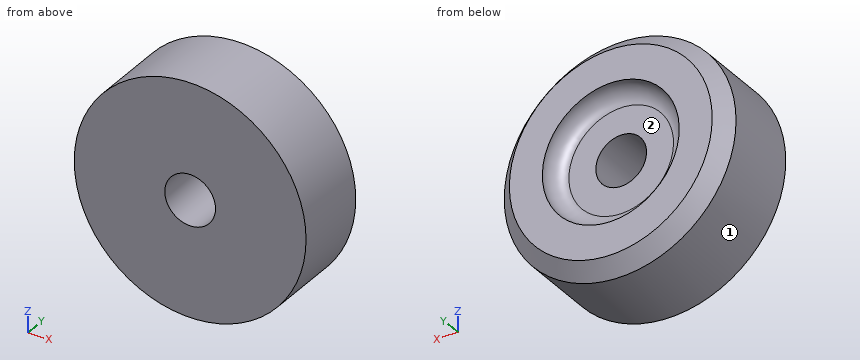
Autodesk Inventor part; units mm, degrees
ref_plane "YZ Plane" through (0, 0, 0) normal (1, 0, 0) x (0, 1, 0)
ref_plane "XZ Plane" through (0, 0, 0) normal (0, 1, 0) x (-1, 0, 0)
ref_plane "XY Plane" through (0, 0, 0) normal (0, 0, 1) x (1, 0, 0)
sketch "Sketch1" plane through (0, 0, 0) normal (0, 0, 1) x (1, 0, 0)
  line L0 (0, 0) -> (0, 6.35)
  line L1 (12.7, 0) -> (0, 0)
  circle A0 centre (10.1178, 6.9428) radius 1.5875
  line L2 (0, 6.35) -> (8.6451, 6.35)
  line L3 (12.7, 0) -> (12.7, 6.35)
  line L4 (12.7, 6.35) -> (11.5905, 6.35)
  line L5 (9.525, 8.4155) -> (0, 8.4155)
  line L6 (0, 8.4155) -> (0, 6.35)
  line L7 (9.525, 8.4155) -> (11.5905, 6.35) construction
  line L8 (9.525, 8.4155) -> (9.525, 10.003)
  line L9 (9.525, 10.003) -> (0, 10.003)
  line L10 (0, 10.003) -> (0, 8.4155)
  line L11 (12.7, 6.35) -> (12.7, 10.003)
  line L12 (12.7, 10.003) -> (9.525, 10.003)
  dimension "d0" = 3.175
  dimension "d5" = 45
  dimension "d6" = 1.5875
  dimension "d7" = 3.175
  dimension "d8" = 6.35
  dimension "d14" = 2.921
  dimension "d37" = 12.7
revolve "Revolution1" add sketch "Sketch1" angle 360 about axis through (0, 10.003, 0) along (0, -1, 0)
sketch "Sketch8" plane through (0, 0, 0) normal (1, 0, 0) x (0, 1, 0)
  circle A0 centre (10.003, -5.734) radius 1.7653
  line L0 (10.003, 0) -> (8.2377, 0)
  line L1 (8.2377, 0) -> (8.2377, -5.734)
  line L2 (10.003, 13.6947) -> (10.003, -13.6947)
  line L3 (10.003, -5.734) -> (10.003, -3.9688) construction
  line L4 (-2.3537, 0) -> (14.1219, 0)
  point P0 (0, 0)
  dimension "d31" = 3.5306
  dimension "d32" = 3.9688
revolve "Revolution3" cut sketch "Sketch8" angle 360 about axis through (0, -10, 0) along (0, 1, 0)
sketch "Sketch9" plane through (0, 8.2377, 0) normal (0, 1, 0) x (1, 0, 0)
  circle A0 centre (0, 0) radius 2.7781
  dimension "d34" = 5.5563
extrude "Extrusion4" cut sketch "Sketch9" against normal through all
chamfer "Chamfer3" distance 1.5875 angle 45 1 edges at (-12.7, 10.003, 0)
properties part number "Diaphragme"
The listing builds one solid part. Answer for the finished solid, in the listing's coordinates (mm). Face numbers are marked on the shaded views. A direction names the side the tool comes from. Give positions to 0.01 mm unless a question says otherwise; leave off trailing zeros. Write each loop counter-clockwise with the first axis right and the second up, starting at its lowest first coordinate (ties: lowest second). Pieces come first, ordered by that corner, then holes. Notation, with made-up numbers: (-2.75, -23) - (4.25, -23) arc R20 cw to (4.25, -4) - close; hole circle Ø6 at (65.25, 66.25). An arc over 180 degrees is marked (long way). Use a Markdown table: item, result.
1. Each of these flat-tipped pins is pushed along its axis until it touches: P1, Ø2, axis at x = 9.5, z = 8, coming from the +Y side; P2, Ø12.5, axis at x = -1.5, z = -1, coming from the +Y side; P3, Ø1.5, axis at y = 8, z = -9, coming from the +X side; P4, Ø2, axis at y = 7.5, z = 6, coming from the -X side. Where does it stop, or does it pass through?
Values follow:
| item | result |
|---|---|
| P1 | stops at y = 9.7 |
| P2 | stops at y = 10 |
| P3 | stops at x = 9.66 |
| P4 | stops at x = -11.67 |
2. Section C-C on y = 1.5 is taken. Write down the section's boundary in (x, z).
Values follow:
| item | result |
|---|---|
| outline | circle Ø25.4 at (0, 0); hole circle Ø5.56 at (0, 0) |
3. Section D-D on y = 9 is taken. Write down the section's boundary in (x, z).
Values follow:
| item | result |
|---|---|
| outline | circle Ø24.23 at (0, 0); hole circle Ø14.37 at (0, 0) |
4. Section A-A on x = 0 is taken. Write down the section's boundary in (y, z).
Values follow:
| item | result |
|---|---|
| outline | (0, -12.7) - (8.42, -12.7) - (10, -11.11) - (10, -7.5) arc R1.77 cw to (8.24, -5.73) - (8.24, -2.78) - (0, -2.78) - close; (0, 2.78) - (8.24, 2.78) - (8.24, 5.73) arc R1.77 cw to (10, 7.5) - (10, 11.11) - (8.42, 12.7) - (0, 12.7) - close |
5. Section B-B on z = 0 is taken. Write down the section's boundary in (x, y).
Values follow:
| item | result |
|---|---|
| outline | (-12.7, 0) - (-2.78, 0) - (-2.78, 8.24) - (-5.73, 8.24) arc R1.77 cw to (-7.5, 10) - (-11.11, 10) - (-12.7, 8.42) - close; (2.78, 0) - (12.7, 0) - (12.7, 8.42) - (11.11, 10) - (7.5, 10) arc R1.77 cw to (5.73, 8.24) - (2.78, 8.24) - close |
6. A tool of negligible diameter and unlimited length cuts with its end or side. For the marked faces 1 and 2, from which of +Z, -Z, +X, -X, +Y, -Y can it reach the whole face along a straight path? Write none if from no direction.
Values follow:
| item | result |
|---|---|
| face 1 | +Y, -Y |
| face 2 | +Y |
7. Find the intervals of material crossed by probe 1 along Z at (x, y) = (0, 2); probe 2 along X at (y, z) = (8.75, -5.5) (3 decimals); probe 3 along X at (y, z) = (7.25, 1.25), in increasing order. Write a range as from..to.
Values follow:
| item | result |
|---|---|
| probe 1 | z = -12.7..-2.78, 2.78..12.7 |
| probe 2 | x = -11.075..-4.294, 4.294..11.075 |
| probe 3 | x = -12.64..-2.48, 2.48..12.64 |
